Part print with two shaded views. Sizes in mm from the minimum x, y, z corner. A direction names the side the tool comes from. Round coordinates to 2 decimals unless told otherwise and drop trailing zeros. Loops run counter-clockwise (first coordinate to the right, second up) from the corner with the lowest first, then second, coordinate; pieces in that order, holes last. Notation, with made-up numbers: (-21, 82) - (-8, 82) arc R8 ccw to (-8, 90) - close; hole circle Ø8 at (31, 16). An arc over 180 degrees is marked (long way). One line per question, with ' | ' between items.
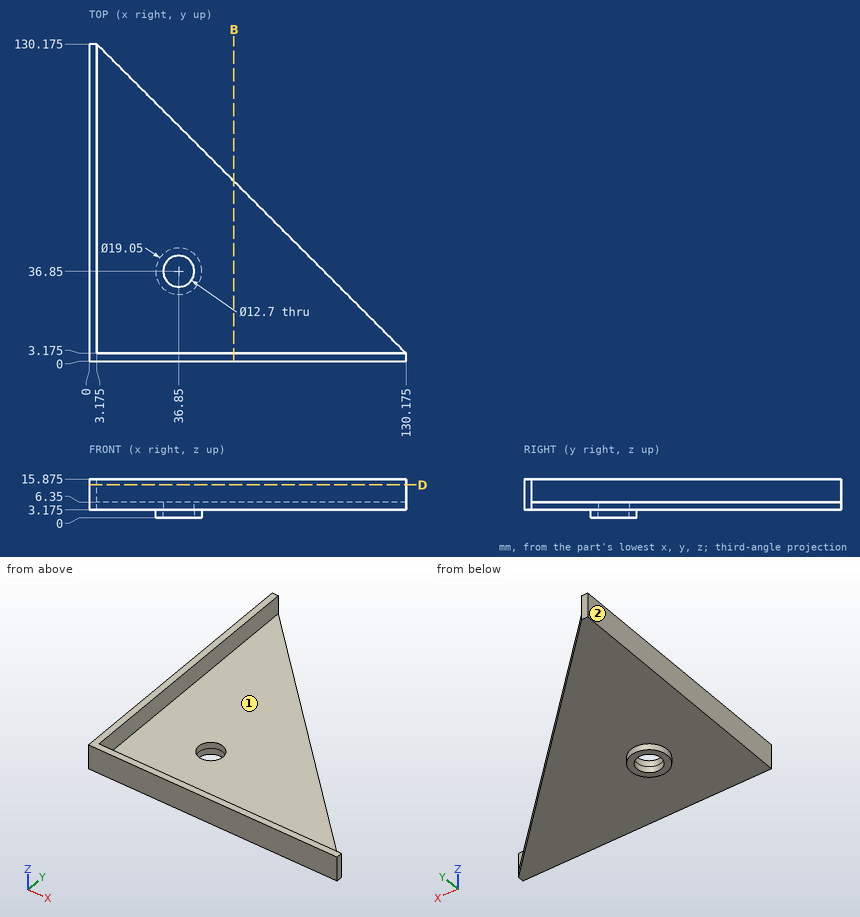
(1) Cut at B-B, the plane x = 59.5. Write the cut outline in (y, z) (3 decimals).
Results found:
outline: (0, 3.175) - (73.85, 3.175) - (73.85, 6.35) - (3.175, 6.35) - (3.175, 15.875) - (0, 15.875) - close
(2) Drop flat-ended pins along their axis: P1, Ø5, axis at x = 74.5, z = 2, coming from the +Y side; P2, Ø3, axis at x = 73.5, z = 13, coming from the +Y side (3 decimals); P3, Ø3, axis at x = 101, z = 2.5, coming from the +Y side; P4, Ø10, axis at x = 36.85, y = 36.85, coming from the -Z side. Give the stop position or say it passes through.
Results found:
P1: stops at y = 61.06 | P2: stops at y = 3.175 | P3: stops at y = 33.69 | P4: passes through
(3) Cut at D-D, the plane z = 13.5. Write the cut outline in (x, y) (3 decimals).
Results found:
outline: (0, 0) - (130.175, 0) - (130.175, 3.175) - (3.175, 3.175) - (3.175, 130.175) - (0, 130.175) - close
(4) Tool access for the marked faces 1 and 2: list every direction of +Z, -Z, +X, -X, +Y, -Y with a clear straight run to the whole face (end or side of a thin tool).
Results found:
face 1: +Z, +X, +Y | face 2: +Z, -Z, -X, +Y, -Y
(5) Probe L1, parallel to Y at x = 46.5, z = 10.5 (3 decimals); L2, parallel to Z at x = 64, y = 52 (3 decimals). List the from-to ranges inside material, lowest first.
Results found:
L1: y = 0 to 3.175 | L2: z = 3.175 to 6.35
